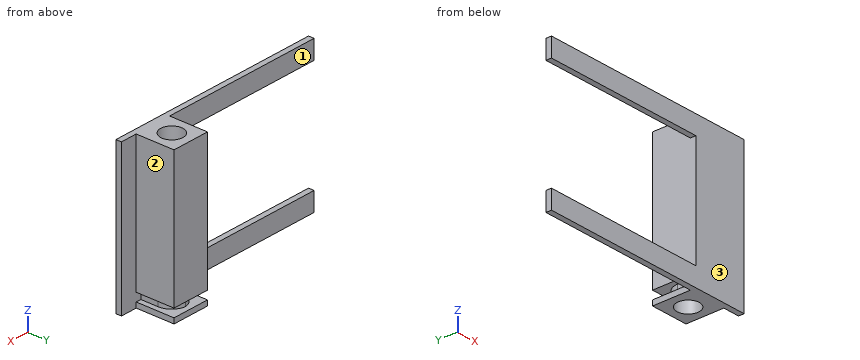
```python
from build123d import *

# Parameters (mm, degrees)
BOSS_EXTRUDE1_DEPTH = 12.7
SKETCH4_W           = 86.8
SKETCH4_H           = 86.8
SKETCH4_R           = 25.4
BOSS_EXTRUDE3_DEPTH = 340
SKETCH6_W           = 86.8
SKETCH6_H           = 19
CUT_EXTRUDE3_DEPTH  = 12
SKETCH7_W           = 19
SKETCH7_H           = 74.8
CUT_EXTRUDE4_DEPTH  = 12
SKETCH8_W           = 19
SKETCH8_H           = 74.8
CUT_EXTRUDE5_DEPTH  = 12
FILLET2_R           = 35


with BuildPart() as part:
    # Sketch1 → Boss-Extrude1 (new body)
    with BuildSketch(Plane(origin=(0, 0, 0), x_dir=(1, 0, 0), z_dir=(0, 1, 0))):
        Polygon((-367.746211961, 196.825353899), (132.253788039, 196.825353899), (132.253788039, -143.174646101), (-367.746211961, -143.174646101), (-367.746211961, -100.174646101), (7.253788039, -100.174646101), (7.253788039, 153.825353899), (-367.746211961, 153.825353899), align=None)
    extrude(amount=BOSS_EXTRUDE1_DEPTH)

    # Sketch4 → Boss-Extrude3 (add)
    with BuildSketch(Plane.XY.offset(143.174646101)):
        with Locations((50.653788039, 56.1)):
            Rectangle(SKETCH4_W, SKETCH4_H)
        with Locations((50.653788039, 56.1)):
            Circle(SKETCH4_R, mode=Mode.SUBTRACT)
    extrude(amount=-BOSS_EXTRUDE3_DEPTH)

    # Sketch6 → Cut-Extrude3 (cut)
    with BuildSketch(Plane(origin=(0, 99.5, 0), x_dir=(1, 0, 0), z_dir=(0, 1, 0))):
        with Locations((50.653788039, 175.325353899)):
            Rectangle(SKETCH6_W, SKETCH6_H)
    extrude(amount=-CUT_EXTRUDE3_DEPTH, mode=Mode.SUBTRACT)

    # Sketch7 → Cut-Extrude4 (cut)
    with BuildSketch(Plane.ZY.offset(-7.253788039)):
        with Locations((-175.325353899, 50.1)):
            Rectangle(SKETCH7_W, SKETCH7_H)
    extrude(amount=-CUT_EXTRUDE4_DEPTH, mode=Mode.SUBTRACT)

    # Sketch8 → Cut-Extrude5 (cut)
    with BuildSketch(Plane(origin=(94.053788039, 0, 0), x_dir=(0, 0, -1), z_dir=(1, 0, 0))):
        with Locations((175.325353899, 50.1)):
            Rectangle(SKETCH8_W, SKETCH8_H)
    extrude(amount=-CUT_EXTRUDE5_DEPTH, mode=Mode.SUBTRACT)

    # Fillet2
    # the kernel refuses this fillet: 35 mm, written as the material it takes off along each edge
    with BuildSketch(Plane(origin=(82.053788039, 87.5, -165.825353899), x_dir=(-1, 0, 0), z_dir=(0, 0, -1))) as fillet2_piece_1:
        with BuildLine():
            CenterArc((FILLET2_R, -FILLET2_R), FILLET2_R, 90, 90)
            Line((0, -FILLET2_R), (0, 0))
            Line((0, 0), (FILLET2_R, 0))
        make_face()
    extrude(amount=19, mode=Mode.SUBTRACT)
    with BuildSketch(Plane(origin=(19.253788039, 87.5, -184.825353899), x_dir=(0, -1, 0), z_dir=(0, 0, 1))) as fillet2_piece_2:
        with BuildLine():
            CenterArc((FILLET2_R, FILLET2_R), FILLET2_R, 180, 90)
            Line((0, FILLET2_R), (0, 0))
            Line((0, 0), (FILLET2_R, 0))
        make_face()
    extrude(amount=19, mode=Mode.SUBTRACT)


solid = part.part
```
Check sheet for the modelled part. Datum: model origin and axes. Units: mm. Face numbers are marked on the shaded views. A direction names the side the tool comes from. Coordinates: 2 decimals unless noted, no trailing zeros. Write each loop counter-clockwise with the first axis right and the second up, starting at its lowest first coordinate (ties: lowest second). Pieces come first, ordered by that corner, then holes. Notation, with made-up numbers: (3, -2.75) - (40, -2.75) arc R28 cw to (40, 34.25) - close; hole circle Ø6 at (62.25, 24.25). An arc over 180 degrees is marked (long way). One line per question, with ' | ' between items.
Item 1: Sectioned sample at C-C on z = -160. Record the boundary of the cut face in (x, y).
Determined:
outline: (-367.75, 0) - (132.25, 0) - (132.25, 12.7) - (94.05, 12.7) - (94.05, 99.5) - (7.25, 99.5) - (7.25, 12.7) - (-367.75, 12.7) - close; hole circle Ø50.8 at (50.65, 56.1)
Item 2: Access from +Z, -Z, +X, -X, +Y, -Y to the whole of each face (thin tool, end or side, straight path). Record for the marked faces 1, 2 and 3.
Determined:
face 1: +Z, -Z, -X, +Y | face 2: +Z, -Z, +X, +Y | face 3: +Z, -Z, +X, -X, -Y
Item 3: Gauge pin test, flat ends, axial feed: P1, Ø15, axis at y = 37.5, z = -177, coming from the +X side; P2, Ø25, axis at x = 113, z = -59.5, coming from the +Y side; P3, Ø6, axis at y = 48.5, z = -188, coming from the +X side. Record the tip position at first contact, or that the pin passes through.
Determined:
P1: stops at x = 82.05 | P2: stops at y = 12.7 | P3: stops at x = 94.05
Item 4: Thickness scan on line 1 (Z direction, x = 84.5, y = 94); line 2 (X direction, y = 56, z = -63); line 3 (Y direction, x = 49.5, z = -135). Record the ranges inside material, lowest first. Write a range as [from, to].
Determined:
line 1: z = [-196.83, -184.83], [-165.83, 143.17] | line 2: x = [7.25, 25.25], [76.05, 94.05] | line 3: y = [0, 30.73], [81.47, 99.5]
Item 5: Sectioned sample at A-A on z = 90. Record the boundary of the cut face in (x, y).
Determined:
outline: (7.25, 0) - (132.25, 0) - (132.25, 12.7) - (94.05, 12.7) - (94.05, 99.5) - (7.25, 99.5) - close; hole circle Ø50.8 at (50.65, 56.1)
Item 6: Sectioned sample at B-B on x = -326. Record the boundary of the cut face in (y, z), plus the area to 3 significant figures.
Determined:
outline: (0, -196.83) - (12.7, -196.83) - (12.7, -153.83) - (0, -153.83) - close; (0, 100.17) - (12.7, 100.17) - (12.7, 143.17) - (0, 143.17) - close | area: 1,090 mm2
